Read the model definition and answer for the solid it produces. Units are mm, in the model's axes. Coordinates: 2 decimals unless noted, no trailing zeros. Write each loop counter-clockwise with the first axis right and the second up, starting at its lowest first coordinate (ties: lowest second). Pieces come first, ordered by that corner, then holes. Notation, with made-up numbers: (24, 22) - (37, 22) arc R24 cw to (37, 33) - close; hole circle Ø2 at (35, 88). An arc over 180 degrees is marked (long way). Use a Markdown table: item, result.
from build123d import *

# Parameters (mm, degrees)
EXTRUDE_1_DEPTH = 50
CHAMFER_1_SIZE  = 0.5
FILLET_1_R      = 0.5


with BuildPart() as part:
    # Эскиз1 → Бобышка-Вытянуть1 (new body)
    with BuildSketch(Plane.XY):
        Polygon((-26.5, 0), (26.5, 0), (26.5, -1.6), (15.2, -6.6), (-15.2, -6.6), (-26.5, -1.6), align=None)
    extrude(amount=EXTRUDE_1_DEPTH)

    # Фаска1
    chamfer_1_edges = [part.edges().sort_by_distance(p)[0] for p in [
        (-26.5, 0, 25),
        (26.5, 0, 25),
        (0, 0, 0),
        (0, 0, 50),
    ]]
    chamfer(chamfer_1_edges, length=CHAMFER_1_SIZE)

    # Скругление1
    fillet_1_edges = [part.edges().sort_by_distance(p)[0] for p in [
        (26.5, -1.6, 25),
        (15.2, -6.6, 25),
        (-15.2, -6.6, 25),
        (-26.5, -1.6, 25),
        (-20.85, -4.1, 50),
        (0, -6.6, 50),
        (20.85, -4.1, 50),
        (20.85, -4.1, 0),
        (0, -6.6, 0),
        (-20.85, -4.1, 0),
    ]]
    fillet(fillet_1_edges, radius=FILLET_1_R)


solid = part.part
(1) Straight lines are drawn through the part: L1, parallel to X at y = -2, z = 15; L2, parallel to X at y = -6, z = 3.5; L3, parallel to Y at x = -17, z = 17.5. For each, find the intervals that lie inside material, in ascending order.
Report:
| item | result |
|---|---|
| L1 | x = -25.6 to 25.6 |
| L2 | x = -16.56 to 16.56 |
| L3 | y = -5.8 to 0 |
(2) Each of these flat-tipped pins is pushed along its axis until it touches: P1, Ø12, axis at x = 17, z = 14.5, coming from the -Y side; P2, Ø2, axis at y = -4, z = 23.5, coming from the -X side. Where does it stop, or does it pass through?
Report:
| item | result |
|---|---|
| P1 | stops at y = -6.6 |
| P2 | stops at x = -23.34 |
(3) A cutting plane is placed at A-A, the plane z = 45.5. Write down the section's boundary in (x, y).
Report:
| item | result |
|---|---|
| outline | (-26.5, -1.27) arc R0.5 ccw to (-26.2, -1.73) - (-15.3, -6.56) arc R0.5 ccw to (-15.09, -6.6) - (15.09, -6.6) arc R0.5 ccw to (15.3, -6.56) - (26.2, -1.73) arc R0.5 ccw to (26.5, -1.27) - (26.5, -0.5) - (26, 0) - (-26, 0) - (-26.5, -0.5) - close |
